The listing builds one solid part. Answer for the finished solid, in the listing's coordinates (mm). Give positions to 0.01 mm unless a question says otherwise; leave off trailing zeros. Write each loop counter-clockwise with the first axis right and the second up, starting at its lowest first coordinate (ties: lowest second). Pieces come first, ordered by that corner, then holes. Notation, with made-up numbers: (38, 22) - (45, 22) arc R16 cw to (45, 44) - close; hole circle Ø1 at (20.5, 7). An arc over 180 degrees is marked (long way). Return JSON: item names as keys, results as strings.
from build123d import *

# Parameters (mm, degrees)
BOSS_EXTRUDE1_DEPTH = 9.525
SKETCH3_R           = 2.0193
CUT_EXTRUDE2_DEPTH  = 10.525


with BuildPart() as part:
    # Sketch1 → Boss-Extrude1 (new body)
    with BuildSketch(Plane(origin=(0, 0, 0), x_dir=(1, 0, 0), z_dir=(0, 1, 0))):
        with BuildLine():
            Line((-10.999999971, -17.78), (10.999999971, -17.78))
            Line((10.999999971, -17.78), (17.349999971, -17.78))
            Line((17.349999971, -17.78), (17.349999971, 0))
            Line((17.349999971, 0), (10.999999971, 0))
            ThreePointArc((10.999999971, 0), (0, -10.999999971), (-10.999999971, 0))
            Line((-10.999999971, 0), (-17.349999971, 0))
            Line((-17.349999971, 0), (-17.349999971, -17.78))
            Line((-17.349999971, -17.78), (-10.999999971, -17.78))
        make_face()
    extrude(amount=BOSS_EXTRUDE1_DEPTH)

    # Sketch3 → Cut-Extrude2 (cut, through all)
    with BuildSketch(Plane(origin=(0, 9.525, 0), x_dir=(1, 0, 0), z_dir=(0, 1, 0))):
        with Locations((11.1125, -11.43)):
            Circle(SKETCH3_R)
        with Locations((-11.1125, -11.43)):
            Circle(SKETCH3_R)
    extrude(amount=-CUT_EXTRUDE2_DEPTH, mode=Mode.SUBTRACT)


solid = part.part
Item 1: The mould has two halves that part along Z. Classify faces 1 (the face through (17.35, 5, 9)), 2 (the face through (12.2, 4.83, 9.73)), 3 (the face through (14, 5, 0)): +Z half, -Z half, draft (parallel to the pull), parting line (faces both ways), or undercut.
Answer below:
{"face 1": "draft", "face 2": "undercut", "face 3": "-Z half"}
Item 2: A cutting plane is placed at B-B on x = 9.5. Determine the outline of the cut face in (y, z) (1 decimal), then the cut area to 3 significant figures.
Answer below:
{"outline": "(0, 5.5) - (9.5, 5.5) - (9.5, 10.2) - (0, 10.2) - close; (0, 12.6) - (9.5, 12.6) - (9.5, 17.8) - (0, 17.8) - close", "area": "93.4 mm²"}
Item 3: Flat-ended cylindrical pins translate along their axes: P1, Ø1.5, axis at x = 2.5, y = 4.5, coming from the -Z side; P2, Ø3, axis at x = 0.5, y = 6, coming from the -Z side. Find the tip coordinate at first contact, or state that the pin passes through.
Answer below:
{"P1": "stops at z = 10.51", "P2": "stops at z = 10.82"}
Item 4: A cutting plane is placed at C-C on y = 8. Determine the outline of the cut face in (x, z), then the cut area to 3 significant figures.
Answer below:
{"outline": "(-17.35, 0) - (-11, 0) arc R11 cw to (11, 0) - (17.35, 0) - (17.35, 17.78) - (-17.35, 17.78) - close; hole circle Ø4.04 at (-11.11, 11.43); hole circle Ø4.04 at (11.11, 11.43)", "area": "401 mm²"}
Item 5: A cutting plane is placed at D-D on z = 6.5. Determine the outline of the cut face in (x, y) (3 decimals).
Answer below:
{"outline": "(-17.35, 0) - (-8.874, 0) - (-8.874, 9.525) - (-17.35, 9.525) - close; (8.874, 0) - (17.35, 0) - (17.35, 9.525) - (8.874, 9.525) - close"}
Item 6: Consider L1, parallel to X at y = 4, z = 11.43; L2, parallel to X at y = 4.25, z = 12.75; L3, parallel to X at y = 6.75, z = 5.5. Determine where each line is inside the solid, lowest interval first.
Answer below:
{"L1": "x = -17.35 to -13.13, -9.09 to 9.09, 13.13 to 17.35", "L2": "x = -17.35 to -12.64, -9.58 to 9.58, 12.64 to 17.35", "L3": "x = -17.35 to -9.53, 9.53 to 17.35"}
Item 7: A cutting plane is placed at A-A on z = 11.43. Determine the outline of the cut face in (x, y) (3 decimals), then the cut area to 3 significant figures.
Answer below:
{"outline": "(-17.35, 0) - (-13.132, 0) - (-13.132, 9.525) - (-17.35, 9.525) - close; (-9.093, 0) - (9.093, 0) - (9.093, 9.525) - (-9.093, 9.525) - close; (13.132, 0) - (17.35, 0) - (17.35, 9.525) - (13.132, 9.525) - close", "area": "254 mm²"}
